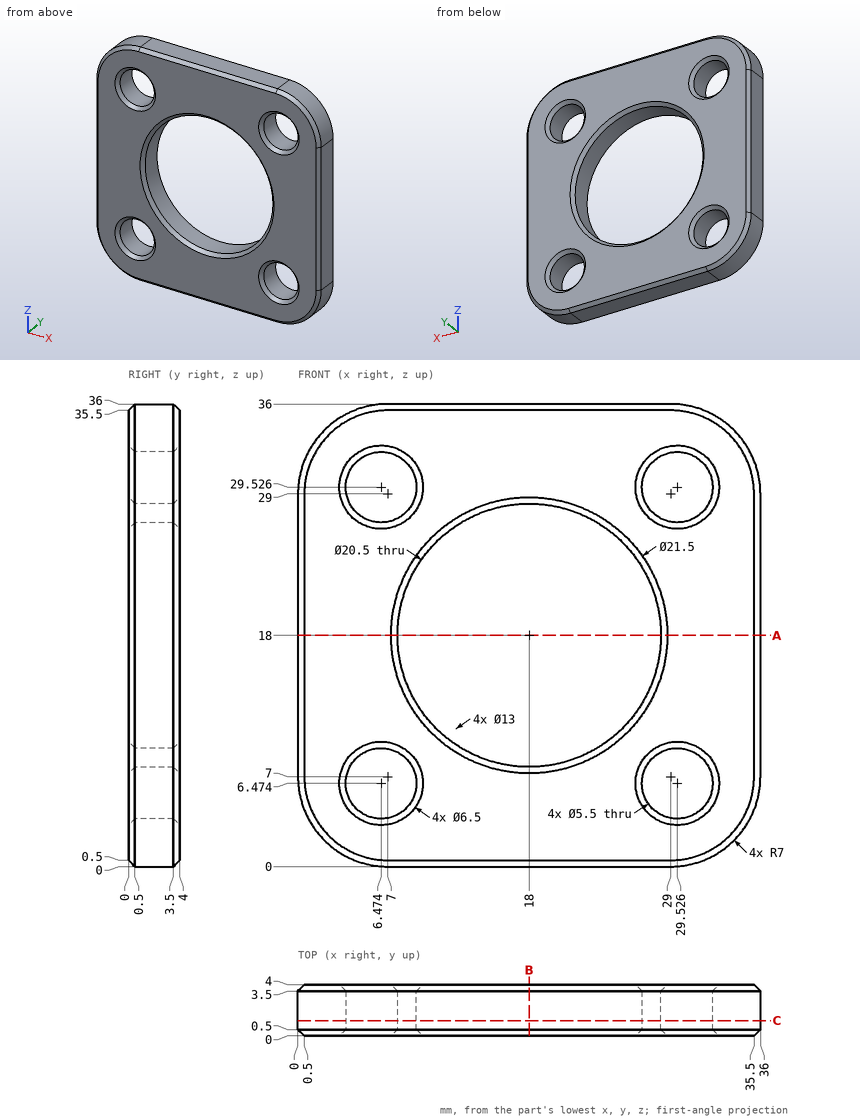
Verification items for this drawing (mm, ordinates from the low corner). Round coordinates to 2 decimals unless told otherwise and drop trailing zeros. Order: outer loops, then holes, each group sorted by start corner. A loop starts at its lowest first (then second) coordinate and runs counter-clockwise, first axis right, second up. Notation, with made-up numbers: M 76,-38 L 105,-38 A21 cw 105,-15 Z; hole C 37,78.5 d9. An arc over 180 degrees is marked long. Answer in a Markdown table with one row per item. Add a question column.
Item 1: Sectioned sample at A-A, the plane z = 18. Enter the section's corners in (x, y).
Item 2: Sectioned sample at C-C, the plane y = 1.2. Enter the section's corners in (x, z).
Item 3: Depth check by flat-ended pin: pin 1 Ø5 at (x, z) = (29.53, 29.53) entering from +Y. Enter the tip coordinate at first touch or a pass-through.
Item 4: Material ranges on L1, parallel to Z at x = 18, y = 1.75; L2, parallel to Z at x = 5, y = 3.45 (1 decimal); L3, parallel to X at y = 3.55, z = 7.5, recorded low to high. Write a range as [from, to].
Item 5: Sectioned sample at B-B, the plane x = 18. Enter the section's corners in (y, z), plus the area to 3 significant figures.
Filled in:
| question | item | result |
|---|---|---|
| 1 | outline | M 0,0.5 L 0.5,0 L 7.25,0 L 7.75,0.5 L 7.75,3.5 L 7.25,4 L 0.5,4 L 0,3.5 Z; M 28.25,0.5 L 28.75,0 L 35.5,0 L 36,0.5 L 36,3.5 L 35.5,4 L 28.75,4 L 28.25,3.5 Z |
| 2 | outline | M 0,7 A7 ccw 7,0 L 29,0 A7 ccw 36,7 L 36,29 A7 ccw 29,36 L 7,36 A7 ccw 0,29 Z; hole C 6.47,6.47 d5.5; hole C 6.47,29.53 d5.5; hole C 18,18 d20.5; hole C 29.53,6.47 d5.5; hole C 29.53,29.53 d5.5 |
| 3 | pin 1 | passes through |
| 4 | L1 | z = [0, 7.75], [28.25, 36] |
| 4 | L2 | z = [0.3, 4.2], [8.8, 27.2], [31.8, 35.7] |
| 4 | L3 | x = [0.05, 3.87], [9.08, 26.92], [32.13, 35.95] |
| 5 | outline | M 0,0.5 L 0.5,0 L 3.5,0 L 4,0.5 L 4,7.25 L 3.5,7.75 L 0.5,7.75 L 0,7.25 Z; M 0,28.75 L 0.5,28.25 L 3.5,28.25 L 4,28.75 L 4,35.5 L 3.5,36 L 0.5,36 L 0,35.5 Z |
| 5 | area | 61.0 mm² |
